from build123d import *

# Parameters (mm, degrees)
SKETCH1_R           = 1.5
BOSS_EXTRUDE1_DEPTH = 5


with BuildPart() as part:
    # Sketch1 → Boss-Extrude1 (new body)
    with BuildSketch(Plane.XY):
        with BuildLine():
            Line((90.09046413, 17.581004237), (128.971852367, 33.226333782))
            ThreePointArc((128.971852367, 33.226333782), (130.33788662, 34.330135362), (130.851957871, 36.009468044))
            Line((130.851957871, 36.009468044), (130.851957871, 39.291849919))
            Line((130.851957871, 39.291849919), (129.683368149, 39.691849919))
            Line((129.683368149, 39.691849919), (127.855440432, 39.291849919))
            Line((127.855440432, 39.291849919), (126.68685071, 39.691849919))
            Line((126.68685071, 39.691849919), (124.858922992, 39.291849919))
            Line((124.858922992, 39.291849919), (123.69033327, 39.691849919))
            Line((123.69033327, 39.691849919), (121.862405553, 39.291849919))
            Line((121.862405553, 39.291849919), (118.330499072, 39.291849919))
            ThreePointArc((118.330499072, 39.291849919), (106.6886691, 38.118374493), (95.046839129, 39.291849919))
            Line((95.046839129, 39.291849919), (94.926233776, 39.291849919))
            Line((94.926233776, 39.291849919), (93.254945284, 39.691849919))
            Line((93.254945284, 39.691849919), (91.761752622, 39.291849919))
            Line((91.761752622, 39.291849919), (90.09046413, 39.691849919))
            Line((90.09046413, 39.691849919), (88.597271468, 39.291849919))
            ThreePointArc((88.597271468, 39.291849919), (85.768844343, 38.120277044), (84.597271468, 35.291849919))
            Line((84.597271468, 35.291849919), (84.597271468, 21.291849919))
            ThreePointArc((84.597271468, 21.291849919), (86.358161226, 17.977278254), (90.09046413, 17.581004237))
        make_face()
        with Locations((88.597271468, 32.460805113)):
            Circle(SKETCH1_R, mode=Mode.SUBTRACT)
        with BuildLine():
            Line((94.167132873, 24.101877808), (94.167132873, 27.719143002))
            ThreePointArc((94.167132873, 27.719143002), (94.313579482, 28.072696393), (94.667132873, 28.219143002))
            Line((94.667132873, 28.219143002), (104.518408295, 28.219143002))
            ThreePointArc((104.518408295, 28.219143002), (105.010688474, 27.806665718), (104.690751088, 27.249783905))
            Line((104.690751088, 27.249783905), (94.839475666, 23.632518711))
            ThreePointArc((94.839475666, 23.632518711), (94.380926126, 23.691895249), (94.167132873, 24.101877808))
        make_face(mode=Mode.SUBTRACT)
        with Locations((115.248465962, 33.15691525)):
            Circle(SKETCH1_R, mode=Mode.SUBTRACT)
        with Locations((125.169093906, 35.649647236)):
            Circle(SKETCH1_R, mode=Mode.SUBTRACT)
        with Locations((98.766505389, 33.15691525)):
            Circle(SKETCH1_R, mode=Mode.SUBTRACT)
        with Locations((106.6886691, 33.15691525)):
            Circle(SKETCH1_R, mode=Mode.SUBTRACT)
        with Locations((88.597271468, 21.291849919)):
            Circle(SKETCH1_R, mode=Mode.SUBTRACT)
    extrude(amount=BOSS_EXTRUDE1_DEPTH)


solid = part.part
Design review of the part built by this model. Coordinates are the model's own, in mm. A direction names the side the tool comes from. Give positions to 0.01 mm unless a question says otherwise; leave off trailing zeros. Write each loop counter-clockwise with the first axis right and the second up, starting at its lowest first coordinate (ties: lowest second). Pieces come first, ordered by that corner, then holes. Notation, with made-up numbers: M -27,-12.75 L 12,-12.75 A22 ccw 12,21.25 Z; hole C -6.75,15 d4. An arc over 180 degrees is marked long. Answer as a JSON object with one key per item and string values. Group by question number.
1) We need section B-B (y = 21.75). Give the boundary of the cut face in (x, z).
2) We need section D-D (x = 116). Give the boundary of the cut face in (y, z).
3) We need section C-C (z = 2.55). Count the separate pieces of the cut face and the enclosed holes in it, and give its area (3 significant figures).
4) Mouldability with a two-part tool opening along X and no side actions: class faces 4 (the face through (85.8, 38.15, 2.46)), 5 (the face through (130.276, 39.489, 2.465)), 6 (the face through (126.6, 36.1, 2.5)) as released by +X, released by -X, zero draft, split by the parting line, or undercut.
5) Tool access review of faces 1 (the face through (94.167, 26, 2)), 2 (the face through (109.259, 25.294, 2.465)), 3 (the face through (90.9, 39.5, 2.5)): name each direction out of +Z, -Z, +X, -X, +Y, -Y from which nothing blocks a thin tool from reaching the whole face with its end or side.
6) For line 1 along X through (y, z) = (34.5, 3.2); line 2 along Y through (x, z) = (103.5, 0.4); line 3 along Y through (x, z) = (114.5, 4.75), list the stretches that pass through material, from the lowest coordinate up.
7) Clearance check with flat-ended pins moving along their axes: pin 1 Ø3 at (y, z) = (32.5, 4.5) entering from +X; pin 2 Ø2 at (x, z) = (90, 0.5) entering from +Y; pin 3 Ø1 at (x, z) = (103.5, 4) entering from -Y; pin 4 Ø1.1 at (y, z) = (25, 2.5) entering from +X. State where each tip first meets the part, or that it passes through.
8) We need section A-A (x = 88). Give the boundary of the cut face in (y, z), and give its area (3 significant figures).
Answer key:
{
 "1": {"outline": "M 84.6,0 L 87.17,0 L 87.17,5 L 84.6,5 Z; M 90.03,0 L 100.45,0 L 100.45,5 L 90.03,5 Z"},
 "2": {"outline": "M 28.01,0 L 31.86,0 L 31.86,5 L 28.01,5 Z; M 34.46,0 L 38.87,0 L 38.87,5 L 34.46,5 Z"},
 "3": {"separate pieces": "1", "enclosed holes": "7", "area": "576 mm²"},
 "4": {"face 4": "released by -X", "face 5": "released by +X", "face 6": "undercut"},
 "5": {"face 1": "+Z, -Z", "face 2": "+Z, -Z, +X, -Y", "face 3": "+Z, -Z, +Y"},
 "6": {"line 1": "x = 84.6 to 98.1, 99.43 to 106.02, 107.36 to 114.58, 115.92 to 124.21, 126.13 to 130.44", "line 2": "y = 22.98 to 26.81, 28.22 to 38.21", "line 3": "y = 27.4 to 31.86, 34.46 to 38.64"},
 "7": {"pin 1": "stops at x = 130.08", "pin 2": "stops at y = 39.69", "pin 3": "stops at y = 22.78", "pin 4": "stops at x = 109.89"},
 "8": {"outline": "M 17.34,0 L 19.92,0 L 19.92,5 L 17.34,5 Z; M 22.67,0 L 31.08,0 L 31.08,5 L 22.67,5 Z; M 33.84,0 L 39.25,0 L 39.25,5 L 33.84,5 Z", "area": "82.0 mm²"}
}
